Verification items for the finished model (mm, model axes). Face numbers are marked on the shaded views. A direction names the side the tool comes from. Coordinates: 2 decimals unless noted, no trailing zeros. Write each loop counter-clockwise with the first axis right and the second up, starting at its lowest first coordinate (ties: lowest second). Pieces come first, ordered by that corner, then holes. Notation, with made-up numbers: M 54,-24.75 L 89,-24.75 A16 cw 89,1.25 Z; hole C -7,20 d6. An arc over 180 degrees is marked long. One line per item, written item: value.
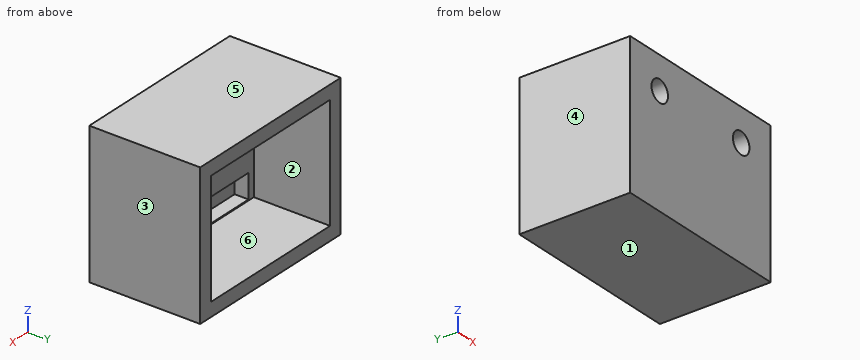
```python
from build123d import *

# Parameters (mm, degrees)
SKETCH1_W           = 20.4
SKETCH1_H           = 16.55
SKETCH1_R           = 1.55
SKETCH1_W_2         = 1
BOSS_EXTRUDE1_DEPTH = 5
SKETCH2_W           = 20.4
SKETCH2_H           = 3.5
CUT_EXTRUDE1_DEPTH  = 2
SKETCH3_W           = 26.4
SKETCH3_H           = 20.55
SKETCH3_W_2         = 22.4
SKETCH3_H_2         = 16.55
BOSS_EXTRUDE2_DEPTH = 16


with BuildPart() as part:
    # Sketch1 → Boss-Extrude1 (new body)
    # profile 1 of 3: a face of its own
    with BuildSketch(Plane(origin=(0, 0, 0), x_dir=(1, 0, 0), z_dir=(0, 1, 0))):
        Rectangle(SKETCH1_W, SKETCH1_H)
        with Locations(Location((-7.65, -5.525, 0), (0, 0, 270))):
            Circle(SKETCH1_R, mode=Mode.SUBTRACT)
        with Locations(Location((7.65, -5.525, 0), (0, 0, 270))):
            Circle(SKETCH1_R, mode=Mode.SUBTRACT)
    # profile 2 of 3: a face of its own
    with BuildSketch(Plane(origin=(0, 0, 0), x_dir=(1, 0, 0), z_dir=(0, 1, 0))):
        with Locations((-10.7, 0)):
            Rectangle(SKETCH1_W_2, SKETCH1_H)
    # profile 3 of 3: a face of its own
    with BuildSketch(Plane(origin=(0, 0, 0), x_dir=(1, 0, 0), z_dir=(0, 1, 0))):
        with Locations((10.7, 0)):
            Rectangle(SKETCH1_W_2, SKETCH1_H)
    extrude(amount=BOSS_EXTRUDE1_DEPTH)

    # Sketch2 → Cut-Extrude1 (cut)
    with BuildSketch(Plane(origin=(0, 5, 0), x_dir=(1, 0, 0), z_dir=(0, 1, 0))):
        with Locations((0, 6.375)):
            Rectangle(SKETCH2_W, SKETCH2_H)
    extrude(amount=-CUT_EXTRUDE1_DEPTH, mode=Mode.SUBTRACT)

    # Sketch3 → Boss-Extrude2 (add)
    with BuildSketch(Plane.XZ):
        Rectangle(SKETCH3_W, SKETCH3_H)
        Rectangle(SKETCH3_W_2, SKETCH3_H_2, mode=Mode.SUBTRACT)
    extrude(amount=-BOSS_EXTRUDE2_DEPTH)


solid = part.part
```
Item 1: Cross-section at C-C, the plane z = -0.25. Enter the section's corners in (x, y).
The answers:
outline: M -13.2,0 L 13.2,0 L 13.2,16 L 11.2,16 L 11.2,5 L -11.2,5 L -11.2,16 L -13.2,16 Z
Item 2: Cross-section at A-A, the plane y = 10.75. Enter the section's corners in (x, z) (3 decimals).
The answers:
outline: M -13.2,-10.275 L 13.2,-10.275 L 13.2,10.275 L -13.2,10.275 Z; hole M -11.2,-8.275 L 11.2,-8.275 L 11.2,8.275 L -11.2,8.275 Z
Item 3: Access from +Z, -Z, +X, -X, +Y, -Y to the whole of each face (thin tool, end or side, straight path). Record for the marked faces 1 and 2.
The answers:
face 1: -Z, +X, -X, +Y, -Y
face 2: +Y
Item 4: Cross-section at D-D, the plane x = 1.25. Enter the section's corners in (y, z) (3 decimals), and give its area (3 significant figures).
The answers:
outline: M 0,-10.275 L 16,-10.275 L 16,-8.275 L 5,-8.275 L 5,-8.125 L 3,-8.125 L 3,-4.625 L 5,-4.625 L 5,8.275 L 16,8.275 L 16,10.275 L 0,10.275 Z
area: 140 mm²
Item 5: Scan lines: line 1 (Z direction, x = -10, y = 12.75) (3 decimals); line 2 (X direction, y = 11.25, z = 3); line 3 (Y direction, x = 1.25, z = 4.25). Record each from-to range of solid material in increasing order.
The answers:
line 1: z = -10.275 to -8.275, 8.275 to 10.275
line 2: x = -13.2 to -11.2, 11.2 to 13.2
line 3: y = 0 to 5
Item 6: Cross-section at B-B, the plane x = -7.65. Enter the section's corners in (y, z) (3 decimals), and give its area (3 significant figures).
The answers:
outline: M 0,-10.275 L 16,-10.275 L 16,-8.275 L 5,-8.275 L 5,-8.125 L 3,-8.125 L 3,-4.625 L 5,-4.625 L 5,3.975 L 0,3.975 Z; M 0,7.075 L 5,7.075 L 5,8.275 L 16,8.275 L 16,10.275 L 0,10.275 Z
area: 124 mm²
Item 7: Go/stop test with a flat-tipped pin: P1, Ø10, axis at x = -2.5, z = 2.5, coming from the +Y side. Record where the tip stops, or that it passes through.
The answers:
P1: stops at y = 5
Item 8: Draft check along X on the marked faces 3, 4, 5 and 6. Enter one of: released by +X, released by -X, zero draft, split by the parting line, or undercut.
The answers:
face 3: released by +X
face 4: released by -X
face 5: zero draft
face 6: undercut
